from build123d import *

# Parameters (mm, degrees)
SKETCH1_R           = 100
BOSS_EXTRUDE1_DEPTH = 100
SKETCH3_R           = 5
BOSS_EXTRUDE2_DEPTH = 10


with BuildPart() as part:
    # Sketch1 → Boss-Extrude1 (new body)
    with BuildSketch(Plane(origin=(0, 0, 0), x_dir=(1, 0, 0), z_dir=(0, 1, 0))):
        Circle(SKETCH1_R)
    extrude(amount=BOSS_EXTRUDE1_DEPTH)

    # Sketch2 → Revolve1 (revolve)
    with BuildSketch(Plane(origin=(0, 0, 0), x_dir=(0, 0, -1), z_dir=(1, 0, 0))):
        Polygon((-100, 0), (-140, 0), (-100, 30), align=None)
    revolve(axis=Axis((0, 0, 0), (0, 1, 0)))

    # Sketch3 → Boss-Extrude2 (add)
    with BuildSketch(Plane(origin=(0, 100, 0), x_dir=(1, 0, 0), z_dir=(0, 1, 0))):
        Circle(SKETCH3_R)
    extrude(amount=BOSS_EXTRUDE2_DEPTH)


solid = part.part
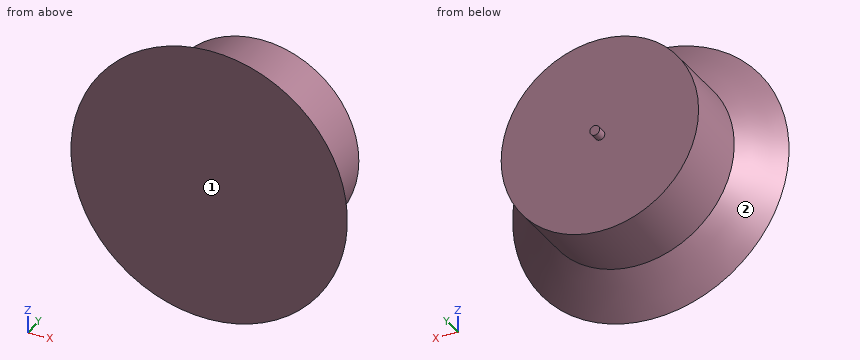
The listing builds one solid part. Answer for the finished solid, in the listing's coordinates (mm). Face numbers are marked on the shaded views. Give positions to 0.01 mm unless a question says otherwise; leave off trailing zeros. Order: outer loops, then holes, each group sorted by start corner. A loop starts at its lowest first (then second) coordinate and runs counter-clockwise, first axis right, second up. Notation, with made-up numbers: (-6, 10.25) - (36, 10.25) arc R14 ccw to (36, 34.25) - close; hole circle Ø7 at (49, -11). An arc over 180 degrees is marked (long way). One line per item, written item: value. Start each with the question number.
1) A cutting plane is placed at A-A on z = 0. Give the vertices of the cut face in (x, y), then the cut area to 3 significant figures.
2) A cutting plane is placed at D-D on y = 78. Give the vertices of the cut face in (x, z), then the cut area to 3 significant figures.
3) Given pin 1 Ø10 at (x, z) = (-16, 97.5) entering from -Y; pin 2 Ø2 at (x, y) = (-50.5, 63) entering from +Z; pin 3 Ø3 at (x, y) = (-16, 85) entering from -Z; pin 4 Ø8 at (x, y) = (-81, 36) entering from -Z, each flat-ended and moving along its own axis, determine where each tip first touches the part or whether it passes through.
4) A cutting plane is placed at B-B on x = 0. Give the vertices of the cut face in (y, z), then the cut area to 3 significant figures.
5) Find the intervals of material crossed by L1, parallel to Y at x = -65.5, z = -55; L2, parallel to Z at x = 66, y = 42; L3, parallel to Y at x = -114, z = -38, in increasing order.
6) The mould has two halves that part along Y. Classify the marked faces 1 and 2: released by +Y, released by -Y, zero draft, split by the parting line, or undercut.
7) A cutting plane is placed at C-C on y = 21. Give the vertices of the cut face in (x, z).
Answer sheet:
1. outline: (-140, 0) - (140, 0) - (100, 30) - (100, 100) - (5, 100) - (5, 110) - (-5, 110) - (-5, 100) - (-100, 100) - (-100, 30) - close
1. area: 21,300 mm2
2. outline: circle Ø200 at (0, 0)
2. area: 31,400 mm2
3. pin 1: stops at y = 0
3. pin 2: stops at z = 86.89
3. pin 3: stops at z = -98.94
3. pin 4: stops at z = -63.8
4. outline: (0, -140) - (30, -100) - (100, -100) - (100, -5) - (110, -5) - (110, 5) - (100, 5) - (100, 100) - (30, 100) - (0, 140) - close
4. area: 21,300 mm2
5. L1: y = 0 to 100
5. L2: z = -75.13 to 75.13
5. L3: y = 0 to 14.88
6. face 1: released by -Y
6. face 2: released by +Y
7. outline: circle Ø224 at (0, 0)
